Geometry check sheet. Reference: the model listing, model coordinates, mm. Coordinates: 2 decimals unless noted, no trailing zeros. Loops run counter-clockwise (first coordinate to the right, second up) from the corner with the lowest first, then second, coordinate; pieces in that order, holes last. Notation, with made-up numbers: (83, 22) -> (90, 22) arc R31 ccw to (90, 58) -> close; hole circle Ø1 at (16.25, -0.5). An arc over 180 degrees is marked (long way). Answer as a JSON object with one key per item and string values.
from build123d import *

# Parameters (mm, degrees)
SKETCH1_W                                      = 306.05
SKETCH1_H                                      = 197.425
SKETCH1_R                                      = 10.775
BOSS_EXTRUDE1_DEPTH                            = 2.38125
SKETCH9_W                                      = 306.05
SKETCH9_H                                      = 2.38125
BOSS_EXTRUDE2_DEPTH                            = 3.175
SKETCH10_R                                     = 3.5
CUT_EXTRUDE1_DEPTH                             = 184.856965146
CSK_FOR_M3_FLAT_HEAD_MACHINE_SCREW1_AT_2_COUNT = 2
CSK_FOR_M3_FLAT_HEAD_MACHINE_SCREW1_AT_2_PITCH = 28.69
CSK_FOR_M3_FLAT_HEAD_MACHINE_SCREW1_AT_3_COUNT = 2
CSK_FOR_M3_FLAT_HEAD_MACHINE_SCREW1_AT_3_PITCH = 83.856540491
CSK_FOR_M3_FLAT_HEAD_MACHINE_SCREW1_AT_4_COUNT = 2
CSK_FOR_M3_FLAT_HEAD_MACHINE_SCREW1_AT_4_PITCH = 178.948509983
CSK_FOR_M3_FLAT_HEAD_MACHINE_SCREW1_AT_5_COUNT = 2
CSK_FOR_M3_FLAT_HEAD_MACHINE_SCREW1_AT_5_PITCH = 208.645558843
CSK_FOR_M3_FLAT_HEAD_MACHINE_SCREW1_AT_6_COUNT = 2
CSK_FOR_M3_FLAT_HEAD_MACHINE_SCREW1_AT_6_PITCH = 260.467597265
CSK_FOR_M3_FLAT_HEAD_MACHINE_SCREW1_AT_7_COUNT = 2
CSK_FOR_M3_FLAT_HEAD_MACHINE_SCREW1_AT_7_PITCH = 272.733119364
CSK_FOR_M3_FLAT_HEAD_MACHINE_SCREW1_AT_8_COUNT = 2
CSK_FOR_M3_FLAT_HEAD_MACHINE_SCREW1_AT_8_PITCH = 224.342
CSK_FOR_M3_FLAT_HEAD_MACHINE_SCREW1_AT_9_COUNT = 2
CSK_FOR_M3_FLAT_HEAD_MACHINE_SCREW1_AT_9_PITCH = 195.652
CSK_FOR_M3_FLAT_HEAD_MACHINE_SCREW1_AT_1_COUNT = 2
CSK_FOR_M3_FLAT_HEAD_MACHINE_SCREW1_AT_1_PITCH = 111.94
SKETCH13_R                                     = 5.999999997
CUT_EXTRUDE2_DEPTH                             = 184.856965146


with BuildPart() as part:
    # Sketch1 → Boss-Extrude1 (new body)
    # profile 1 of 5: a face of its own
    with BuildSketch(Plane.XY):
        Rectangle(SKETCH1_W, SKETCH1_H)
        with Locations((-142.25, -87.9375)):
            Circle(SKETCH1_R, mode=Mode.SUBTRACT)
        with Locations((-130.25, -64.9375)):
            Circle(SKETCH1_R, mode=Mode.SUBTRACT)
    # profile 2 of 5: a face of its own
    with BuildSketch(Plane.XY):
        with Locations((-130.25, -64.9375)):
            Circle(SKETCH1_R)
    # profile 3 of 5: a face of its own
    with BuildSketch(Plane.XY):
        with Locations((-142.25, -87.9375)):
            Circle(SKETCH1_R)
    # profile 4 of 5: a face of its own
    with BuildSketch(Plane.XY):
        with BuildLine():
            ThreePointArc((-142.25, -98.7125), (-149.869075567, -95.556575567), (-153.025, -87.9375))
            Line((-153.025, -87.9375), (-153.025, -98.7125))
            Line((-153.025, -98.7125), (-142.25, -98.7125))
        make_face()
    # profile 5 of 5: a face of its own
    with BuildSketch(Plane.XY):
        Rectangle(SKETCH1_W, SKETCH1_H)
    extrude(amount=BOSS_EXTRUDE1_DEPTH)

    # Sketch9 → Boss-Extrude2 (add)
    with BuildSketch(Plane(origin=(0, 98.7125, 0), x_dir=(1, 0, 0), z_dir=(0, 1, 0))):
        with Locations((0, -1.190625)):
            Rectangle(SKETCH9_W, SKETCH9_H)
    extrude(amount=BOSS_EXTRUDE2_DEPTH)

    # Sketch10 → Cut-Extrude1 (cut, through all)
    with BuildSketch(Plane(origin=(0, 0, 0), x_dir=(-1, 0, 0), z_dir=(0, 0, -1))):
        with Locations((-134.610000066, 92.362499989)):
            Circle(SKETCH10_R)
        with Locations((-124.450000066, 92.362499989)):
            Circle(SKETCH10_R)
        with Locations((-143.817500066, -87.537500111)):
            Circle(SKETCH10_R)
        with Locations((-133.657500066, -87.537500111)):
            Circle(SKETCH10_R)
    cut_extrude1 = extrude(amount=-CUT_EXTRUDE1_DEPTH, mode=Mode.SUBTRACT)

    # Mirror1: Cut-Extrude1 across plane
    add(cut_extrude1.mirror(Plane(origin=(0, 0, 0), x_dir=(0, 0, 1), z_dir=(1, 0, 0))), mode=Mode.SUBTRACT)

    # Sketch12 → CSK for M3 Flat Head Machine Screw1 (revolve, cut)
    with BuildSketch(Plane(origin=(111.94, -83.7125, 0), x_dir=(0, 1, 0), z_dir=(1, 0, 0))):
        Polygon((0, 0), (0, 2.38125), (1.7, 2.38125), (1.7, 1.45), (3.15, 0), align=None)
    csk_for_m3_flat_head_machine_screw1 = revolve(axis=Axis((111.94, -83.7125, -6.35), (0, 0, 1)), mode=Mode.SUBTRACT)

    # CSK for M3 Flat Head Machine Screw1 at 2: CSK for M3 Flat Head Machine Screw1 ×2
    with Locations(*[(-i * CSK_FOR_M3_FLAT_HEAD_MACHINE_SCREW1_AT_2_PITCH, 0, 0) for i in range(1, CSK_FOR_M3_FLAT_HEAD_MACHINE_SCREW1_AT_2_COUNT)]):
        add(csk_for_m3_flat_head_machine_screw1, mode=Mode.SUBTRACT)

    # CSK for M3 Flat Head Machine Screw1 at 3: CSK for M3 Flat Head Machine Screw1 ×2
    with Locations(*[Vector(0.34281762477474764, 0.9394019779326636, 0) * (i * CSK_FOR_M3_FLAT_HEAD_MACHINE_SCREW1_AT_3_PITCH) for i in range(1, CSK_FOR_M3_FLAT_HEAD_MACHINE_SCREW1_AT_3_COUNT)]):
        add(csk_for_m3_flat_head_machine_screw1, mode=Mode.SUBTRACT)

    # CSK for M3 Flat Head Machine Screw1 at 4: CSK for M3 Flat Head Machine Screw1 ×2
    with Locations(*[Vector(-0.17848709666882537, 0.9839422525345344, 0) * (i * CSK_FOR_M3_FLAT_HEAD_MACHINE_SCREW1_AT_4_PITCH) for i in range(1, CSK_FOR_M3_FLAT_HEAD_MACHINE_SCREW1_AT_4_COUNT)]):
        add(csk_for_m3_flat_head_machine_screw1, mode=Mode.SUBTRACT)

    # CSK for M3 Flat Head Machine Screw1 at 5: CSK for M3 Flat Head Machine Screw1 ×2
    with Locations(*[Vector(-0.5365079449598532, 0.8438952689729663, 0) * (i * CSK_FOR_M3_FLAT_HEAD_MACHINE_SCREW1_AT_5_PITCH) for i in range(1, CSK_FOR_M3_FLAT_HEAD_MACHINE_SCREW1_AT_5_COUNT)]):
        add(csk_for_m3_flat_head_machine_screw1, mode=Mode.SUBTRACT)

    # CSK for M3 Flat Head Machine Screw1 at 6: CSK for M3 Flat Head Machine Screw1 ×2
    with Locations(*[Vector(-0.7369054808176366, 0.6759957931384839, 0) * (i * CSK_FOR_M3_FLAT_HEAD_MACHINE_SCREW1_AT_6_PITCH) for i in range(1, CSK_FOR_M3_FLAT_HEAD_MACHINE_SCREW1_AT_6_COUNT)]):
        add(csk_for_m3_flat_head_machine_screw1, mode=Mode.SUBTRACT)

    # CSK for M3 Flat Head Machine Screw1 at 7: CSK for M3 Flat Head Machine Screw1 ×2
    with Locations(*[Vector(-0.9262809761508288, 0.37683358823367613, 0) * (i * CSK_FOR_M3_FLAT_HEAD_MACHINE_SCREW1_AT_7_PITCH) for i in range(1, CSK_FOR_M3_FLAT_HEAD_MACHINE_SCREW1_AT_7_COUNT)]):
        add(csk_for_m3_flat_head_machine_screw1, mode=Mode.SUBTRACT)

    # CSK for M3 Flat Head Machine Screw1 at 8: CSK for M3 Flat Head Machine Screw1 ×2
    with Locations(*[(-i * CSK_FOR_M3_FLAT_HEAD_MACHINE_SCREW1_AT_8_PITCH, 0, 0) for i in range(1, CSK_FOR_M3_FLAT_HEAD_MACHINE_SCREW1_AT_8_COUNT)]):
        add(csk_for_m3_flat_head_machine_screw1, mode=Mode.SUBTRACT)

    # CSK for M3 Flat Head Machine Screw1 at 9: CSK for M3 Flat Head Machine Screw1 ×2
    with Locations(*[(-i * CSK_FOR_M3_FLAT_HEAD_MACHINE_SCREW1_AT_9_PITCH, 0, 0) for i in range(1, CSK_FOR_M3_FLAT_HEAD_MACHINE_SCREW1_AT_9_COUNT)]):
        add(csk_for_m3_flat_head_machine_screw1, mode=Mode.SUBTRACT)

    # CSK for M3 Flat Head Machine Screw1 at 1: CSK for M3 Flat Head Machine Screw1 ×2
    with Locations(*[(-i * CSK_FOR_M3_FLAT_HEAD_MACHINE_SCREW1_AT_1_PITCH, 0, 0) for i in range(1, CSK_FOR_M3_FLAT_HEAD_MACHINE_SCREW1_AT_1_COUNT)]):
        add(csk_for_m3_flat_head_machine_screw1, mode=Mode.SUBTRACT)

    # Sketch13 → Cut-Extrude2 (cut, through all)
    with BuildSketch(Plane(origin=(0, 0, 0), x_dir=(-1, 0, 0), z_dir=(0, 0, -1))):
        with Locations((-97.75, -79.7125001)):
            Circle(SKETCH13_R)
        with Locations((97.75, -79.7125001)):
            Circle(SKETCH13_R)
    extrude(amount=-CUT_EXTRUDE2_DEPTH, mode=Mode.SUBTRACT)


solid = part.part
1. Section check A-A, the plane x = 97.75. Record the boundary of the cut face in (y, z), then the cut area to 3 significant figures.
Evaluation:
{"outline": "(-98.71, 0) -> (-85.71, 0) -> (-85.71, 2.38) -> (-98.71, 2.38) -> close; (-73.71, 0) -> (101.89, 0) -> (101.89, 2.38) -> (-73.71, 2.38) -> close", "area": "449 mm^2"}
2. Thickness scan on probe 1 along Y at (x, z) = (-97.75, 0.85); probe 2 along X at (y, z) = (-88, 1.25) (3 decimals); probe 3 along Y at (x, z) = (-124.45, 1.6). Record the ranges inside material, lowest first. Write a range as from..to.
Evaluation:
{"probe 1": "y = -98.71..-85.71, -73.71..101.89", "probe 2": "x = -153.025..-147.287, -140.348..-137.127, -130.188..130.188, 137.127..140.348, 147.287..153.025", "probe 3": "y = -98.71..88.86, 95.86..101.89"}
3. Depth check by flat-ended pin: P1, Ø5.5, axis at x = -140.69, y = 19.06, coming from the +Z side; P2, Ø5.5, axis at x = 80, y = 92.36, coming from the -Z side. Enter the tip coordinate at first touch or a pass-through.
Evaluation:
{"P1": "stops at z = 2.38", "P2": "stops at z = 0.4"}
4. Mould release check, pull along Y, two halves, no side actions. Record for faces 1 (the face through (-2, 0, 0)), 2 (the face through (140.48, -86.49, 1.17)): released by +Y, released by -Y, zero draft, split by the parting line, or undercut.
Evaluation:
{"face 1": "zero draft", "face 2": "undercut"}
